from build123d import *

# Parameters (mm, degrees)
SKETCH1_W           = 101.6
SKETCH1_H           = 76.2
BOSS_EXTRUDE1_DEPTH = 6.35
SKETCH2_W           = 6.35
SKETCH2_H           = 19.05
BOSS_EXTRUDE2_DEPTH = 31.75
SKETCH3_R           = 4.7625
CUT_EXTRUDE1_DEPTH  = 116.003391254
FILLET1_R           = 3.175
FILLET2_R           = 9.525
CHAMFER1_SIZE       = 44.45


with BuildPart() as part:
    # Sketch1 → Boss-Extrude1 (new body)
    with BuildSketch(Plane(origin=(0, 0, 0), x_dir=(1, 0, 0), z_dir=(0, 1, 0))):
        Rectangle(SKETCH1_W, SKETCH1_H)
    extrude(amount=BOSS_EXTRUDE1_DEPTH)

    # Sketch2 → Boss-Extrude2 (add)
    with BuildSketch(Plane(origin=(0, 6.35, 0), x_dir=(1, 0, 0), z_dir=(0, 1, 0))):
        with Locations((-47.625, -28.575)):
            Rectangle(SKETCH2_W, SKETCH2_H)
        with Locations((-28.575, -28.575)):
            Rectangle(SKETCH2_W, SKETCH2_H)
        with Locations((28.575, 28.575)):
            Rectangle(SKETCH2_W, SKETCH2_H)
        with Locations((47.625, 28.575)):
            Rectangle(SKETCH2_W, SKETCH2_H)
    extrude(amount=BOSS_EXTRUDE2_DEPTH)

    # Sketch3 → Cut-Extrude1 (cut, through all)
    with BuildSketch(Plane(origin=(50.8, 0, 0), x_dir=(0, 0, -1), z_dir=(1, 0, 0))):
        with Locations((28.575, 28.575)):
            Circle(SKETCH3_R)
        with Locations((-28.575, 28.575)):
            Circle(SKETCH3_R)
    extrude(amount=-CUT_EXTRUDE1_DEPTH, mode=Mode.SUBTRACT)

    # Fillet1
    fillet1_edges = [part.edges().sort_by_distance(p)[0] for p in [
        (-47.625, 6.35, 19.05),
        (-28.575, 6.35, 19.05),
        (28.575, 6.35, -19.05),
        (47.625, 6.35, -19.05),
    ]]
    fillet(fillet1_edges, radius=FILLET1_R)

    # Fillet2
    fillet2_edges = [part.edges().sort_by_distance(p)[0] for p in [
        (28.575, 38.1, -38.1),
        (47.625, 38.1, -38.1),
        (-47.625, 38.1, 19.05),
        (-47.625, 38.1, 38.1),
        (-28.575, 38.1, 19.05),
        (-28.575, 38.1, 38.1),
        (28.575, 38.1, -19.05),
        (47.625, 38.1, -19.05),
    ]]
    fillet(fillet2_edges, radius=FILLET2_R - 0.0001)  # a hair under: the kernel refuses the full size

    # Chamfer1
    chamfer1_edges = [part.edges().sort_by_distance(p)[0] for p in [
        (-50.8, 3.175, -38.1),
        (50.8, 3.175, 38.1),
    ]]
    chamfer(chamfer1_edges, length=CHAMFER1_SIZE)


solid = part.part
Input: part model. Units: mm. Frame: model coordinates. A direction names the side the tool comes from. Give positions to 0.01 mm unless a question says otherwise; leave off trailing zeros. Loops run counter-clockwise (first coordinate to the right, second up) from the corner with the lowest first, then second, coordinate; pieces in that order, holes last. Notation, with made-up numbers: (-9, 85) - (47, 85) arc R20 ccw to (47, 94) - close; hole circle Ø2 at (20.25, 9). An arc over 180 degrees is marked (long way). Use CSV: the item, a comma, the result in double quotes. Start each with the question number.
Item 1: Contact query for flat-ended pins moving along their axis: P1, Ø8, axis at x = -15.5, y = 8, coming from the +Z side; P2, Ø5, axis at x = 28, y = 18, coming from the +Z side; P3, Ø18, axis at y = 19, z = -26, coming from the -X side; P4, Ø7, axis at x = -29, y = 22.5, coming from the -Z side. Output: stop coordinate, or through.
Item 2: Line query: line 1 (X direction, y = 34, z = -22); line 2 (X direction, y = 21, z = 20); line 3 (Y direction, x = 10, z = 25.5). Output: solid intervals per line, ascending.
Item 3: Section C-C on z = 21. Return loops of the section in (x, y), then the cut area to 3 significant figures.
Item 4: Mould query, pull axis Y, two halves, no side actions, for faces 4 (the cylindrical face through (-28.531, 23.926, 29.607)), 5 (the flat face through (-1, 6.35, -1)), 6 (the flat face through (-28.26, 3.13, -16.19)). Classes: pulls with the +Y half, pulls with the -Y half, needs draft (parallel to the pull), parting line crosses it, or undercut.
Item 5: Section A-A on y = 26. State how many separate pieces and enclosed holes the cut face has, then the cut area to 3 significant figures.
Item 6: Reachability of faces 1 (the flat face through (-48, 19, 19.05)), 2 (the flat face through (44.45, 18, -29)), 3 (the flat face through (29, 19, -19.05)) from +Z, -Z, +X, -X, +Y, -Y: full face, straight path, thin tool, end or side. Return the list, or none.
Ans:
1,P1,"stops at z = 38.1"
1,P2,"stops at z = -19.05"
1,P3,"stops at x = 25.4"
1,P4,"stops at z = 19.05"
2,line 1,"x = 25.4 to 31.75, 44.45 to 50.8"
2,line 2,"x = -50.8 to -44.45, -31.75 to -25.4"
2,line 3,"y = 0 to 6.35"
3,outline,"(-50.8, 0) - (23.45, 0) - (23.45, 6.35) - (-25.4, 6.35) - (-25.4, 34.35) - (-31.75, 34.35) - (-31.75, 6.35) - (-44.45, 6.35) - (-44.45, 34.35) - (-50.8, 34.35) - close"
3,area,"827 mm2"
4,face 4,"undercut"
4,face 5,"pulls with the +Y half"
4,face 6,"needs draft"
5,separate pieces,"8"
5,enclosed holes,"0"
5,area,"280 mm2"
6,face 1,"-Z, +X, -X, +Y"
6,face 2,"+Z, -Z, +Y"
6,face 3,"+Z, +X, -X, +Y"
